Could you check a few things on this drawing? It's one solid part, dimensions in mm from its lowest x, y, z. Round coordinates to 2 decimals unless told otherwise and drop trailing zeros. Loops run counter-clockwise (first coordinate to the right, second up) from the corner with the lowest first, then second, coordinate; pieces in that order, holes last. Notation, with made-up numbers: M 70.25,5 L 128.25,5 A16 ccw 128.25,31 Z; hole C -20,-16 d9. An arc over 180 degrees is marked long. Put each result on its own line as item: value. Start each with the question number.
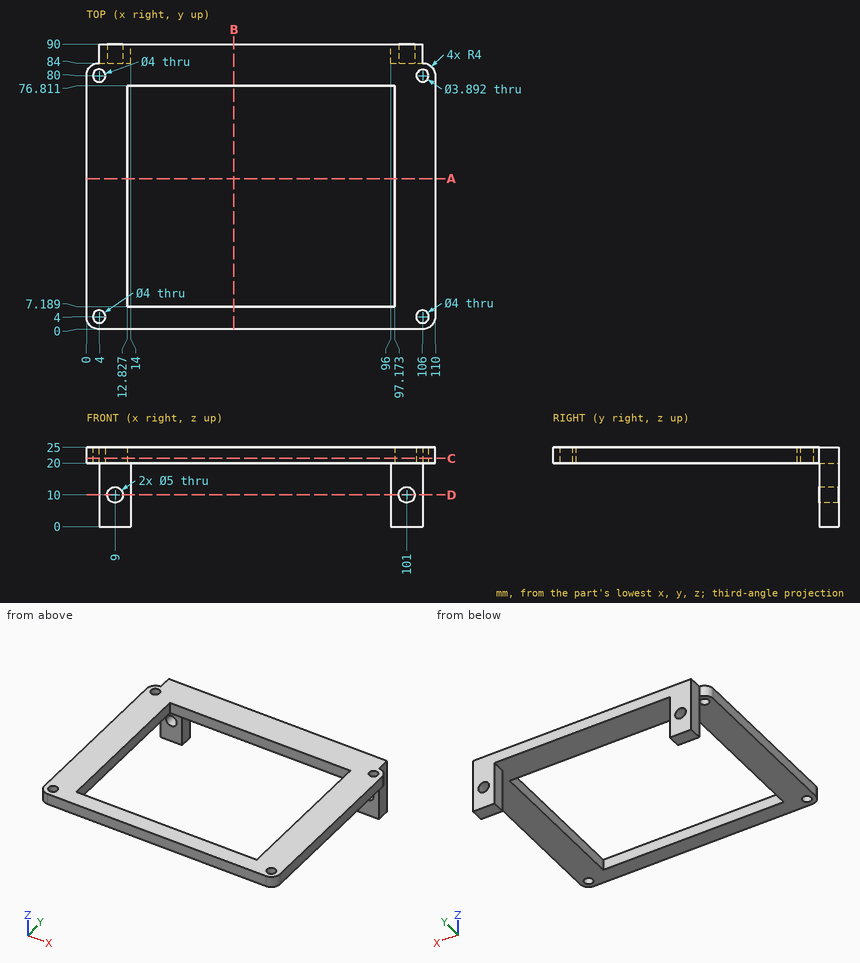
1) Suppose I cut it at D-D (z = 10). Write out the boundary of the cut face in (x, y), plus the area to 3 significant figures.
2) I'm going to push flat-ended pins straight in: P1, Ø3, axis at y = 85.5, z = 12, coming from the -X side; P2, Ø11, axis at x = 7, z = 13.5, coming from the -Y side; P3, Ø5, axis at y = 88.5, z = 8.5, coming from the +X side; P4, Ø12, axis at y = 40.5, z = 18, coming from the -X side. Where does each tip first touch, or does it pass through?
3) If I drill on probe 1 along X at (y, z) = (87.6, 10); probe 2 along X at (y, z) = (10, 21.75); probe 3 along Y at (x, z) = (34, 21.75), over which ranges is the centre line in solid material (lowest first)? Write a range as from..to.
4) Suppose I cut it at B-B (x = 46.5). Write out the boundary of the cut face in (y, z).
5) Suppose I cut it at C-C (z = 21.5). Write out the boundary of the cut face in (x, y), plus the area to 3 significant figures.
6) Suppose I cut it at A-A (y = 47.5). Write out the boundary of the cut face in (x, z), plus the area to 3 significant figures.
Results are:
1. outline: M 4,84 L 6.5,84 L 6.5,90 L 4,90 Z; M 11.5,84 L 14,84 L 14,90 L 11.5,90 Z; M 96,84 L 98.5,84 L 98.5,90 L 96,90 Z; M 103.5,84 L 106,84 L 106,90 L 103.5,90 Z
1. area: 60.0 mm²
2. P1: x = 4
2. P2: y = 84
2. P3: x = 106
2. P4: x = 0
3. probe 1: 4..6.5, 11.5..14, 96..98.5, 103.5..106
3. probe 2: 0..12.83, 97.17..110
3. probe 3: 0..7.19, 76.81..90
4. outline: M 0,20 L 7.19,20 L 7.19,25 L 0,25 Z; M 76.81,20 L 90,20 L 90,25 L 76.81,25 Z
5. outline: M 0,4 A4 ccw 4,0 L 106,0 A4 ccw 110,4 L 110,80 A4 ccw 106,84 L 106,90 L 4,90 L 4,84 A4 ccw 0,80 Z; hole C 4,4 d4; hole C 4,80 d4; hole M 12.83,7.19 L 97.17,7.19 L 97.17,76.81 L 12.83,76.81 Z; hole C 106,4 d4; hole C 106,80 d3.89
5. area: 3,920 mm²
6. outline: M 0,20 L 12.83,20 L 12.83,25 L 0,25 Z; M 97.17,20 L 110,20 L 110,25 L 97.17,25 Z
6. area: 128 mm²
